from build123d import *

# Parameters (mm, degrees)
EXTRUDE_1_DEPTH = 254
SKETCH_3_R      = 25
EXTRUDE_2_DEPTH = 2.5
CHAMFER_1_SIZE  = 3


with BuildPart() as part:
    # 草图2 → 凸台-拉伸1 (new body)
    with BuildSketch(Plane.XY):
        with BuildLine():
            Line((6, 4), (6, -4))
            ThreePointArc((6, -4), (0, -10), (-6, -4))
            Line((-6, -4), (-6, 4))
            ThreePointArc((-6, 4), (0, 10), (6, 4))
        make_face()
    extrude(amount=EXTRUDE_1_DEPTH)

    # 草图3 → 凸台-拉伸2 (add)
    with BuildSketch(Plane.XY.offset(254)):
        Circle(SKETCH_3_R)
    extrude(amount=EXTRUDE_2_DEPTH)

    # 倒角1
    chamfer_1_edges = [part.edges().sort_by_distance(p)[0] for p in [
        (0, -10, 254),
        (6, 0, 254),
        (0, 10, 254),
        (-6, 0, 254),
    ]]
    chamfer(chamfer_1_edges, length=CHAMFER_1_SIZE)

    # 草图4 → 旋转1 (revolve)
    with BuildSketch(Plane(origin=(0, 0, 0), x_dir=(0, 0, -1), z_dir=(1, 0, 0))):
        with BuildLine():
            Line((-256.5, 0), (-256.5, -19.669640386))
            ThreePointArc((-256.5, -19.669640386), (-268.52081528, -14.690455667), (-273.5, -2.669640386))
            Line((-273.5, -2.669640386), (-273.5, 0))
            Line((-273.5, 0), (-256.5, 0))
        make_face()
    revolve(axis=Axis((0, 0, 273.5), (0, 0, -1)))


solid = part.part
Could you check a few things on this model? Use its own coordinates, in mm. A direction names the side the tool comes from. Give positions to 0.01 mm unless a question says otherwise; leave off trailing zeros. Write each loop counter-clockwise with the first axis right and the second up, starting at its lowest first coordinate (ties: lowest second). Pieces come first, ordered by that corner, then holes. Notation, with made-up numbers: (51.5, 5) -> (71.5, 5) arc R16 ccw to (71.5, 25) -> close; hole circle Ø6 at (18.5, 57). An arc over 180 degrees is marked (long way). Write each question's results on one line, items separated by ' | '. Start each with the question number.
Q1. I need wall thicknesses on probe 1 along X at (y, z) = (-3, 112.5); probe 2 along Z at (x, y) = (-14, 15); probe 3 along Y at (x, z) = (-4.5, 20.5). Which ranges of each line are inside material? Lowest first, please.
Q2. Which directions (+Z, -Z, +X, -X, +Y, -Y) give clear straight access to the entire face, cutting with the end or side of a thin tool? Please do faces 1 (the face through (0, -10, 124)), 2 (the face through (-6, 0, 124)), 3 (the face through (0, 10, 124)), 4 (the face through (-15, -13, 256.5)), 5 (the face through (6, 0, 124)).
Q3. I'm going to push flat-ended pins straight in: pin 1 Ø2.5 at (y, z) = (1, 112.5) entering from -X; pin 2 Ø10 at (x, z) = (7.5, 76) entering from -Y; pin 3 Ø4 at (x, y) = (18.5, 12.5) entering from +Z; pin 4 Ø25 at (x, y) = (-0.5, 11.5) entering from +Z. Where does each tip first touch, or does it pass through?
Q4. Suppose I cut it at A-A, the plane z = 245. List the corners of the cut face in (x, y) for me.
Outcome:
1) probe 1: -6 to 6 | probe 2: 254 to 256.5 | probe 3: -7.97 to 7.97
2) face 1: -Z, -Y | face 2: -Z, -X, +Y, -Y | face 3: -Z, +Y | face 4: +Z | face 5: -Z, +X, +Y, -Y
3) pin 1: x = -6 | pin 2: y = -9.45 | pin 3: z = 256.5 | pin 4: z = 273.5
4) outline: (-6, -4) arc R6 ccw to (6, -4) -> (6, 4) arc R6 ccw to (-6, 4) -> close
